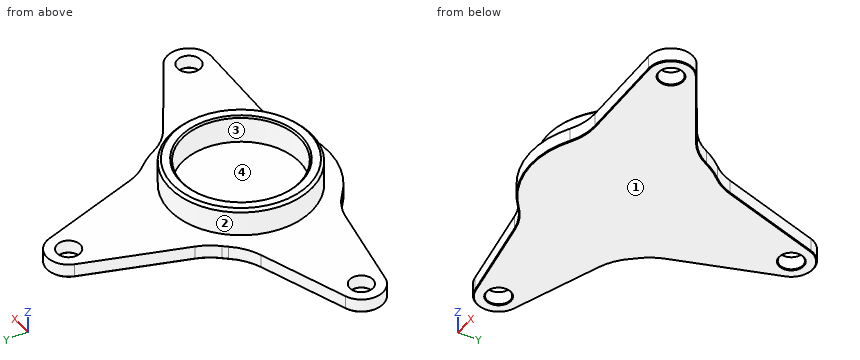
from build123d import *

# Parameters (mm, degrees)
ESQUISSE1_R        = 25.985
ESQUISSE1_R_2      = 21.5
BOSS_EXTRU_1_DEPTH = 10
CHANFREIN1_SIZE    = 1
CHANFREIN2_SIZE    = 0.6
ESQUISSE2_R        = 4.25
BOSS_EXTRU_2_DEPTH = 5
CHANFREIN3_SIZE    = 0.25


with BuildPart() as part:
    # Esquisse1 → Boss.-Extru.1 (new body)
    with BuildSketch(Plane.XY):
        Circle(ESQUISSE1_R)
        Circle(ESQUISSE1_R_2, mode=Mode.SUBTRACT)
    extrude(amount=BOSS_EXTRU_1_DEPTH)

    # Chanfrein1
    chanfrein1_edges = [part.edges().sort_by_distance(p)[0] for p in [
        (-25.985, 0, 10),
    ]]
    chamfer(chanfrein1_edges, length=CHANFREIN1_SIZE)

    # Chanfrein2
    chanfrein2_edges = [part.edges().sort_by_distance(p)[0] for p in [
        (-21.5, 0, 10),
    ]]
    chamfer(chanfrein2_edges, length=CHANFREIN2_SIZE)

    # Esquisse2 → Boss.-Extru.2 (add)
    with BuildSketch(Plane(origin=(0, 0, 0), x_dir=(-1, 0, 0), z_dir=(0, 0, -1))):
        with BuildLine():
            Line((7.60845213, 65.472135955), (19.562751949, 28.680584205))
            ThreePointArc((19.562751949, 28.680584205), (21.2719439, 24.846095602), (23.743927554, 21.452876365))
            ThreePointArc((23.743927554, 21.452876365), (24.442816498, 20.653055987), (25.114776372, 19.830481783))
            ThreePointArc((25.114776372, 19.830481783), (29.077787425, 16.028245766), (33.925593306, 13.447309217))
            Line((33.925593306, 13.447309217), (65.50114543, 1.86803233))
            ThreePointArc((65.50114543, 1.86803233), (70.71462295, -6.359410431), (64.116870777, -13.524661891))
            Line((64.116870777, -13.524661891), (30.982002055, -19.284490011))
            ThreePointArc((30.982002055, -19.284490011), (25.751494228, -20.959077483), (21.173682289, -23.993231927))
            ThreePointArc((21.173682289, -23.993231927), (3.185198765, -31.841082093), (-16.001386984, -27.712012099))
            ThreePointArc((-16.001386984, -27.712012099), (-21.089512057, -25.644782414), (-26.548088017, -25.039469423))
            Line((-26.548088017, -25.039469423), (-60.167318575, -25.957337556))
            ThreePointArc((-60.167318575, -25.957337556), (-68.053671575, -20.240992693), (-64.573244793, -11.143861737))
            Line((-64.573244793, -11.143861737), (-35.917071141, 6.460650663))
            ThreePointArc((-35.917071141, 6.460650663), (-31.676574653, 9.950728723), (-28.545263087, 14.462639983))
            ThreePointArc((-28.545263087, 14.462639983), (-26.377181723, 18.117513195), (-23.743927554, 21.452876365))
            ThreePointArc((-23.743927554, 21.452876365), (-21.2719439, 24.846095602), (-19.562751949, 28.680584205))
            Line((-19.562751949, 28.680584205), (-7.60845213, 65.472135955))
            ThreePointArc((-7.60845213, 65.472135955), (0, 71), (7.60845213, 65.472135955))
        make_face()
        with Locations((0, 63)):
            Circle(ESQUISSE2_R, mode=Mode.SUBTRACT)
        with Locations((62.746778111, -5.642857143)):
            Circle(ESQUISSE2_R, mode=Mode.SUBTRACT)
        with Locations((-60.385652242, -17.96031746)):
            Circle(ESQUISSE2_R, mode=Mode.SUBTRACT)
    extrude(amount=BOSS_EXTRU_2_DEPTH)

    # Chanfrein3
    chanfrein3_edges = [part.edges().sort_by_distance(p)[0] for p in [
        (-25.751494228, -20.959077483, -5),
        (-47.549436416, -16.404575951, -5),
        (-70.71462295, -6.359410431, -5),
        (-49.713369368, 7.657670773, -5),
        (-29.077787425, 16.028245766, -5),
        (-24.442816498, 20.653055987, -5),
        (-21.2719439, 24.846095602, -5),
        (-13.58560204, 47.07636008, -5),
        (0, 71, -5),
        (13.58560204, 47.07636008, -5),
        (21.2719439, 24.846095602, -5),
        (26.377181723, 18.117513195, -5),
        (31.676574653, 9.950728723, -5),
        (50.245157967, -2.341605537, -5),
        (68.053671575, -20.240992693, -5),
        (43.357703296, -25.498403489, -5),
        (21.089512057, -25.644782414, -5),
        (-3.185198765, -31.841082093, -5),
        (4.25, 63, -5),
        (-58.496778111, -5.642857143, -5),
        (64.635652242, -17.96031746, -5),
    ]]
    chamfer(chanfrein3_edges, length=CHANFREIN3_SIZE)


solid = part.part
The model under review builds one solid part; all positions refer to its coordinate system, in mm. Face numbers are marked on the shaded views. Round coordinates to 2 decimals unless told otherwise and drop trailing zeros. Loops run counter-clockwise (first coordinate to the right, second up) from the corner with the lowest first, then second, coordinate; pieces in that order, holes last. Notation, with made-up numbers: M 80,79.5 L 138,79.5 A27 cw 138,100.5 Z; hole C -34,87.25 d10. An arc over 180 degrees is marked long. Answer as CSV lines item,"result". Start each with the question number.
Item 1: Wall thickness on line 1 (Z direction, x = 48.5, y = -8); line 2 (Y direction, x = 58.5, z = -2); line 3 (X direction, y = 7, z = 8.75): over which ranges is each line inside the solid? List them lowest first. Write a range as [from, to].
Item 2: Consider section A-A (x = 0). Write out the cut boundary in (y, z) (3 decimals).
Item 3: Consider section C-C (z = 2). Write out the cut boundary in (x, y) (3 decimals), then the cut area to 3 significant figures.
Item 4: Mouldability with a two-part tool opening along X and no side actions: class the marked faces 1, 2, 3 and 4 as released by +X, released by -X, zero draft, split by the parting line, or undercut.
Item 5: Insertion check: P1, Ø5, axis at x = -62.75, y = -5.64, coming from the -Z side; P2, Ø3, axis at x = 49.5, y = -7.5, coming from the +Z side; P3, Ø8, axis at x = 16.5, z = 8.5, coming from the +Y side; P4, Ø1, axis at x = -20.5, z = 6, coming from the +Y side. Each pin has a flat end and moves straight along its axis. Give the tip position at first contact, or say it passes through.
Item 6: Consider section D-D (x = -50.5). Write out the cut boundary in (y, z).
Item 7: Consider section B-B (y = 63). Write out the cut boundary in (x, z).
Answer:
1,line 1,"z = [-5, 0]"
1,line 2,"y = [-25.91, -21.77], [-14.15, -7.41]"
1,line 3,"x = [-25.02, -20.33], [20.33, 25.02]"
2,outline,"M -32,-4.75 L -31.75,-5 L 58.5,-5 L 58.75,-4.75 L 58.75,0 L 25.985,0 L 25.985,9 L 24.985,10 L 22.1,10 L 21.5,9.4 L 21.5,0 L -21.5,0 L -21.5,9.4 L -22.1,10 L -24.985,10 L -25.985,9 L -25.985,0 L -32,0 Z; M 67.25,-4.75 L 67.5,-5 L 70.75,-5 L 71,-4.75 L 71,0 L 67.25,0 Z"
3,outline,"C 0,0 d51.97; hole C 0,0 d43"
3,area,"669 mm^2"
4,face 1,"zero draft"
4,face 2,"split by the parting line"
4,face 3,"undercut"
4,face 4,"undercut"
5,P1,"passes through"
5,P2,"stops at z = 0"
5,P3,"stops at y = 22.78"
5,P4,"stops at y = 16.59"
6,outline,"M -15.89,-4.75 L -15.64,-5 L 7.1,-5 L 7.37,-4.75 L 7.37,0 L -15.89,0 Z"
7,outline,"M -8.41,-4.75 L -8.15,-5 L -4.5,-5 L -4.25,-4.75 L -4.25,0 L -8.41,0 Z; M 4.25,-4.75 L 4.5,-5 L 8.15,-5 L 8.41,-4.75 L 8.41,0 L 4.25,0 Z"
